The listing builds one solid part. Answer for the finished solid, in the listing's coordinates (mm). Round coordinates to 2 decimals unless told otherwise and drop trailing zeros. Loops run counter-clockwise (first coordinate to the right, second up) from the corner with the lowest first, then second, coordinate; pieces in that order, holes last. Notation, with made-up numbers: M 58.25,24 L 82.25,24 A18 cw 82.25,37 Z; hole C -30.75,-29 d1. An arc over 180 degrees is marked long. Answer as a JSON object with one key per item and string values.
```python
from build123d import *

# Parameters (mm, degrees)
F0_R     = 47.5
F0_R_2   = 3.75
F0_R_3   = 32.5
F1_DEPTH = 5


with BuildPart() as f1:
    # F0 (on Top) → F1 (new body)
    with BuildSketch(Plane.XY):
        Circle(F0_R)
        with Locations((0, -39.861098)):
            Circle(F0_R_2, mode=Mode.SUBTRACT)
        with Locations((-40.148903, 0)):
            Circle(F0_R_2, mode=Mode.SUBTRACT)
        Circle(F0_R_3, mode=Mode.SUBTRACT)
        with Locations((39.573293, 0)):
            Circle(F0_R_2, mode=Mode.SUBTRACT)
        with Locations((0, 40.148903)):
            Circle(F0_R_2, mode=Mode.SUBTRACT)
    extrude(amount=-F1_DEPTH)


solid = f1.part
```
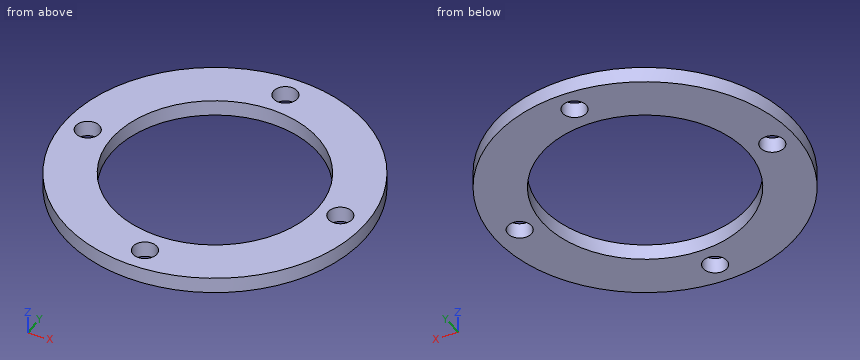
Item 1: The part is cut by section A-A (y = -19). Give the vertices of the cut face in (x, z), then the cut area to 3 significant figures.
Values follow:
{"outline": "M -43.53,-5 L -26.37,-5 L -26.37,0 L -43.53,0 Z; M 26.37,-5 L 43.53,-5 L 43.53,0 L 26.37,0 Z", "area": "172 mm^2"}
Item 2: Flat-ended cylindrical pins translate along their axes: P1, Ø3, axis at x = -20.5, z = -1.5, coming from the +Y side; P2, Ø1.5, axis at y = -20.5, z = -2.5, coming from the -X side; P3, Ø8, axis at x = 26, y = 0.5, coming from the +Z side; P4, Ø1.5, axis at y = -15.5, z = -4, coming from the -X side. Find the tip coordinate at first contact, or state that the pin passes through.
Values follow:
{"P1": "y = 43.53", "P2": "x = -43.2", "P3": "through", "P4": "x = -45.15"}
Item 3: The part is cut by section D-D (z = -1.75). Give the vertices of the cut face in (x, y).
Values follow:
{"outline": "C 0,0 d95; hole C -40.15,0 d7.5; hole C 0,0 d65; hole C 0,-39.86 d7.5; hole C 0,40.15 d7.5; hole C 39.57,0 d7.5"}
Item 4: The part is cut by section B-B (x = -38). Give the vertices of the cut face in (y, z).
Values follow:
{"outline": "M -28.5,-5 L -3.07,-5 L -3.07,0 L -28.5,0 Z; M 3.07,-5 L 28.5,-5 L 28.5,0 L 3.07,0 Z"}
Item 5: Straight lines are drawn through the part: line 1 (Y direction, x = 0, z = -1.55); line 2 (Y direction, x = 41, z = -2.35); line 3 (X direction, y = 0.5, z = -3.85). For each, find the intervals that lie inside material, in ascending order.
Values follow:
{"line 1": "-47.5 to -43.61, -36.11 to -32.5, 32.5 to 36.4, 43.9 to 47.5", "line 2": "-23.98 to -3.47, 3.47 to 23.98", "line 3": "-47.5 to -43.87, -36.43 to -32.5, 32.5 to 35.86, 43.29 to 47.5"}
Item 6: The part is cut by section C-C (y = 0). Give the vertices of the cut face in (x, z), then the cut area to 3 significant figures.
Values follow:
{"outline": "M -47.5,-5 L -43.9,-5 L -43.9,0 L -47.5,0 Z; M -36.4,-5 L -32.5,-5 L -32.5,0 L -36.4,0 Z; M 32.5,-5 L 35.82,-5 L 35.82,0 L 32.5,0 Z; M 43.32,-5 L 47.5,-5 L 47.5,0 L 43.32,0 Z", "area": "75.0 mm^2"}
